Print and shaded views of the part. All mm, measured from the part's lowest x, y and z. Round coordinates to 2 decimals unless told otherwise and drop trailing zeros. Loops run counter-clockwise (first coordinate to the right, second up) from the corner with the lowest first, then second, coordinate; pieces in that order, holes last. Notation, with made-up numbers: (78, 64.5) -> (121, 64.5) arc R15 ccw to (121, 81.5) -> close; hole circle Ø9 at (46, -20). An arc over 180 degrees is marked (long way). Answer as CSV lines item,"result".
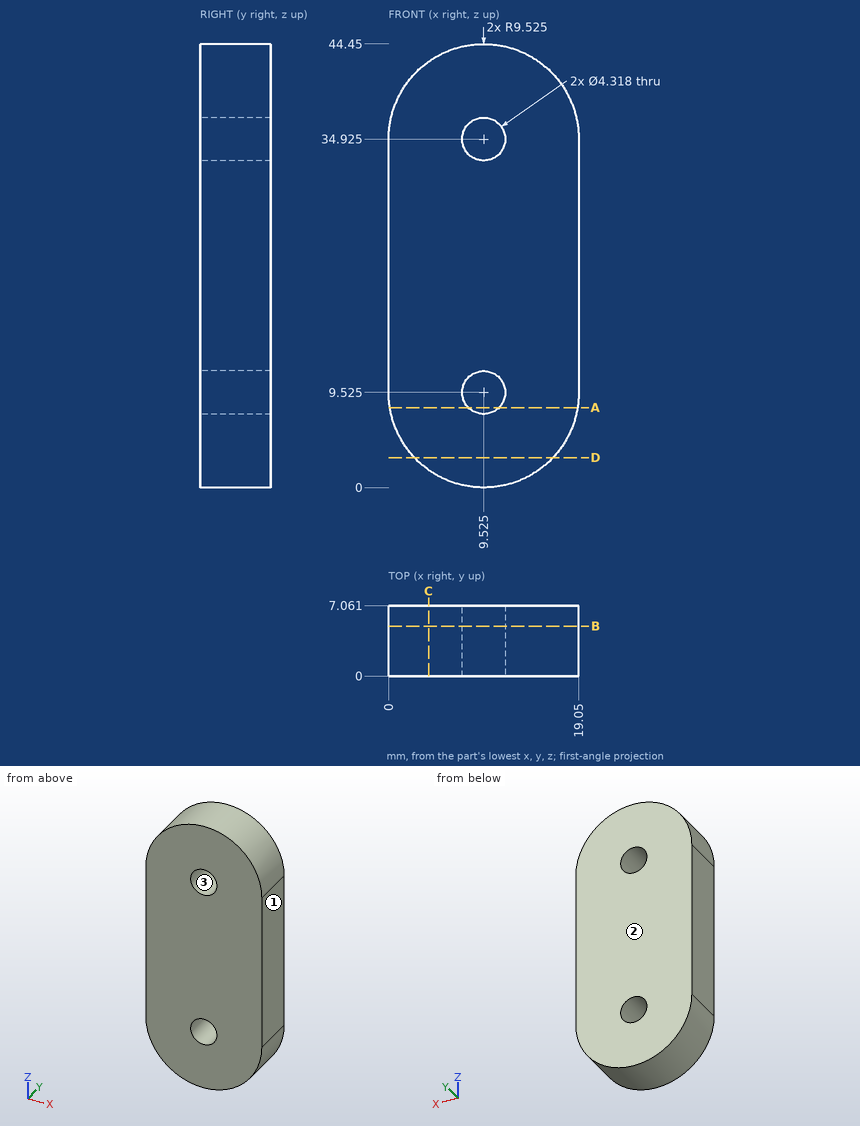
Q1. Slice it at A-A, the plane z = 8. Give the cut face in (x, y).
Results:
outline,"(0.12, 0) -> (8, 0) -> (8, 7.06) -> (0.12, 7.06) -> close; (11.05, 0) -> (18.93, 0) -> (18.93, 7.06) -> (11.05, 7.06) -> close"
Q2. Slice it at B-B, the plane y = 5. Give the cut face in (x, z) (3 decimals).
Results:
outline,"(0, 9.525) arc R9.525 ccw to (19.05, 9.525) -> (19.05, 34.925) arc R9.525 ccw to (0, 34.925) -> close; hole circle Ø4.318 at (9.525, 9.525); hole circle Ø4.318 at (9.525, 34.925)"
Q3. Drop flat-ended pins along their axis: pin 1 Ø1 at (x, y) = (11.5, 5) entering from +Z; pin 2 Ø3 at (y, z) = (4.5, 39.5) entering from +X. Give the stop position or say it passes through.
Results:
pin 1,"z = 44.34"
pin 2,"x = 18.54"
Q4. Two-plate mould, pull along X, no slides. Class the marked faces 1, 2 and 3: pulls with the +X half, pulls with the -X half, needs draft (parallel to the pull), parting line crosses it, or undercut.
Results:
face 1,"pulls with the +X half"
face 2,"needs draft"
face 3,"undercut"
Q5. Slice it at C-C, the plane x = 4. Give the cut face in (y, z), and give its area (3 significant figures).
Results:
outline,"(0, 1.77) -> (7.06, 1.77) -> (7.06, 42.68) -> (0, 42.68) -> close"
area,"289 mm2"
Q6. Slice it at D-D, the plane z = 3. Give the cut face in (x, y), and give its area (3 significant figures).
Results:
outline,"(2.59, 0) -> (16.46, 0) -> (16.46, 7.06) -> (2.59, 7.06) -> close"
area,"98.0 mm2"
Q7. Probe L1, parallel to Z at x = 8.5, y = 5.25; L2, parallel to Z at x = 8.75, y = 4.5; L3, parallel to X at y = 3.25, z = 35. List the from-to ranges inside material, lowest first. Write a range as [from, to].
Results:
L1,"[0.06, 7.62], [11.43, 33.02], [36.83, 44.39]"
L2,"[0.03, 7.51], [11.54, 32.91], [36.94, 44.42]"
L3,"[0, 7.37], [11.68, 19.05]"
